Design review of the part built by this model. Coordinates are the model's own, in mm. A direction names the side the tool comes from. Round coordinates to 2 decimals unless told otherwise and drop trailing zeros. Loops run counter-clockwise (first coordinate to the right, second up) from the corner with the lowest first, then second, coordinate; pieces in that order, holes last. Notation, with made-up numbers: (-15.75, -31) -> (-0.75, -31) arc R13 ccw to (-0.75, -16) -> close; hole circle Ø3 at (58, -23.75). An arc over 180 degrees is marked (long way). Use a Markdown table: item, result. Add a question column.
from build123d import *
from build123d.topology import SkipClean

# Parameters (mm, degrees)
SKETCH1_R           = 2.875
SKETCH1_W           = 55.75
SKETCH1_H           = 3.25
BOSS_EXTRUDE1_DEPTH = 3.25
SKETCH1_4_W         = 55.75
SKETCH1_4_H         = 3.25
BOSS_EXTRUDE2_DEPTH = 40
CUT_EXTRUDE2_DEPTH  = 43.25
BOSS_EXTRUDE4_DEPTH = 2
BOSS_EXTRUDE5_DEPTH = 43.25
SKETCH2_R           = 5
SKETCH2_R_2         = 2.875
CUT_EXTRUDE1_DEPTH  = 17.25
FILLET1_R           = 1
SKETCH2_3_R         = 5
SKETCH2_3_R_2       = 2.875
BOSS_EXTRUDE6_DEPTH = 3.25
SKETCH4_R           = 1.5
CUT_EXTRUDE4_DEPTH  = 45.25
FILLET4_R           = 1
FILLET5_R           = 10


# Some blends are built 0.0001 mm under size
with BuildPart() as part:
    # Sketch1 → Boss-Extrude1 (new body)
    # profile 1 of 2: a face of its own
    with BuildSketch(Plane.XY):
        Polygon((-17.875, -10), (37.875, -10), (37.875, -6.375), (37.875, 26.375), (-17.875, 26.375), (-17.875, -6.375), align=None)
        with Locations(Location((20, 20, 0), (0, 0, 180))):
            Circle(SKETCH1_R, mode=Mode.SUBTRACT)
        with Locations(Location((20, 0, 0), (0, 0, 180))):
            Circle(SKETCH1_R, mode=Mode.SUBTRACT)
        with Locations(Location((0, 0, 0), (0, 0, 180))):
            Circle(SKETCH1_R, mode=Mode.SUBTRACT)
        with Locations(Location((0, 20, 0), (0, 0, 180))):
            Circle(SKETCH1_R, mode=Mode.SUBTRACT)
    # profile 2 of 2: a face of its own
    with BuildSketch(Plane.XY):
        with Locations((10, -11.625)):
            Rectangle(SKETCH1_W, SKETCH1_H)
    extrude(amount=BOSS_EXTRUDE1_DEPTH)

    # Sketch1<4> → Boss-Extrude2 (add)
    with BuildSketch(Plane.XY):
        with Locations((10, -11.625)):
            Rectangle(SKETCH1_4_W, SKETCH1_4_H)
    extrude(amount=-BOSS_EXTRUDE2_DEPTH)

    # Sketch3 → Cut-Extrude2 (cut)
    with BuildSketch(Plane.XY.offset(3.25)):
        with BuildLine():
            Line((12.253469547, -13.25), (7.746530453, -13.25))
            ThreePointArc((7.746530453, -13.25), (7.84573728, -20.807857289), (14.375, -17))
            ThreePointArc((14.375, -17), (13.807857289, -14.84573728), (12.253469547, -13.25))
        make_face()
        with BuildLine():
            ThreePointArc((12.253469547, -13.25), (10, -12.625), (7.746530453, -13.25))
            Line((7.746530453, -13.25), (12.253469547, -13.25))
        make_face()
    extrude(amount=-CUT_EXTRUDE2_DEPTH, mode=Mode.SUBTRACT)

    # Sketch3<4> → Boss-Extrude4 (add)
    with BuildSketch(Plane.XY.offset(3.25)):
        Polygon((3.793484606, -13.25), (-17.875, -13.25), (-17.875, -27.25), (37.875, -27.25), (37.875, -13.25), (16.206515394, -13.25), (18.371578903, -17), (14.185789452, -24.25), (5.814210548, -24.25), (1.628421097, -17), align=None)
        Polygon((37.875, -6.75), (-17.875, -6.75), (-17.875, -13.25), (3.793484606, -13.25), (5.814210548, -9.75), (14.185789452, -9.75), (16.206515394, -13.25), (37.875, -13.25), align=None)
    extrude(amount=BOSS_EXTRUDE4_DEPTH)

    # Sketch3<5> → Boss-Extrude5 (add)
    with SkipClean():  # the faces are left unmerged after this step: merging them gives an invalid solid
        with BuildSketch(Plane.XY.offset(3.25)):
            Polygon((3.793484606, -13.25), (-17.875, -13.25), (-17.875, -27.25), (37.875, -27.25), (37.875, -13.25), (16.206515394, -13.25), (18.371578903, -17), (14.185789452, -24.25), (5.814210548, -24.25), (1.628421097, -17), align=None)
            with BuildLine():
                Line((7.746530453, -13.25), (3.793484606, -13.25))
                Line((3.793484606, -13.25), (1.628421097, -17))
                Line((1.628421097, -17), (5.814210548, -24.25))
                Line((5.814210548, -24.25), (14.185789452, -24.25))
                Line((14.185789452, -24.25), (18.371578903, -17))
                Line((18.371578903, -17), (16.206515394, -13.25))
                Line((16.206515394, -13.25), (12.253469547, -13.25))
                ThreePointArc((12.253469547, -13.25), (13.807857289, -14.84573728), (14.375, -17))
                ThreePointArc((14.375, -17), (7.84573728, -20.807857289), (7.746530453, -13.25))
            make_face()
        extrude(amount=-BOSS_EXTRUDE5_DEPTH)

    # Sketch2 → Cut-Extrude1 (cut)
    # profile 1 of 8: a face of its own
    with SkipClean():  # the faces are left unmerged after this step: merging them gives an invalid solid
        with BuildSketch(Plane.XZ.offset(10)):
            with Locations(Location((20, -10, 0), (0, 0, 90))):
                Circle(SKETCH2_R)
            with Locations((20, -10)):
                Circle(SKETCH2_R_2, mode=Mode.SUBTRACT)
        # profile 2 of 8: a face of its own
        with BuildSketch(Plane.XZ.offset(10)):
            with Locations((20, -10)):
                Circle(SKETCH2_R_2)
        # profile 3 of 8: a face of its own
        with BuildSketch(Plane.XZ.offset(10)):
            with Locations(Location((0, -10, 0), (0, 0, 90))):
                Circle(SKETCH2_R)
            with Locations((0, -10)):
                Circle(SKETCH2_R_2, mode=Mode.SUBTRACT)
        # profile 4 of 8: a face of its own
        with BuildSketch(Plane.XZ.offset(10)):
            with Locations((0, -10)):
                Circle(SKETCH2_R_2)
        # profile 5 of 8: a face of its own
        with BuildSketch(Plane.XZ.offset(10)):
            with Locations(Location((0, -30, 0), (0, 0, 90))):
                Circle(SKETCH2_R)
            with Locations((0, -30)):
                Circle(SKETCH2_R_2, mode=Mode.SUBTRACT)
        # profile 6 of 8: a face of its own
        with BuildSketch(Plane.XZ.offset(10)):
            with Locations((0, -30)):
                Circle(SKETCH2_R_2)
        # profile 7 of 8: a face of its own
        with BuildSketch(Plane.XZ.offset(10)):
            with Locations(Location((20, -30, 0), (0, 0, 90))):
                Circle(SKETCH2_R)
            with Locations((20, -30)):
                Circle(SKETCH2_R_2, mode=Mode.SUBTRACT)
        # profile 8 of 8: a face of its own
        with BuildSketch(Plane.XZ.offset(10)):
            with Locations((20, -30)):
                Circle(SKETCH2_R_2)
        extrude(amount=CUT_EXTRUDE1_DEPTH, mode=Mode.SUBTRACT)

    # Fillet1
    fillet1_edges = [part.edges().sort_by_distance(p)[0] for p in [
        (10, -6.75, 3.25),
    ]]
    fillet(fillet1_edges, radius=FILLET1_R)
    fillet1_2_edges = [part.edges().sort_by_distance(p)[0] for p in [
        (10, -6.75, 5.25),
    ]]
    fillet(fillet1_2_edges, radius=FILLET1_R - 0.0001)  # a hair under: the kernel refuses the full size

    # Sketch2<3> → Boss-Extrude6 (add)
    # profile 1 of 4: a face of its own
    with BuildSketch(Plane.XZ.offset(10)):
        with Locations(Location((20, -10, 0), (0, 0, 90))):
            Circle(SKETCH2_3_R)
        with Locations(Location((20, -10, 0), (0, 0, 90))):
            Circle(SKETCH2_3_R_2, mode=Mode.SUBTRACT)
    # profile 2 of 4: a face of its own
    with BuildSketch(Plane.XZ.offset(10)):
        with Locations(Location((0, -10, 0), (0, 0, 90))):
            Circle(SKETCH2_3_R)
        with Locations(Location((0, -10, 0), (0, 0, 90))):
            Circle(SKETCH2_3_R_2, mode=Mode.SUBTRACT)
    # profile 3 of 4: a face of its own
    with BuildSketch(Plane.XZ.offset(10)):
        with Locations(Location((0, -30, 0), (0, 0, 90))):
            Circle(SKETCH2_3_R)
        with Locations(Location((0, -30, 0), (0, 0, 90))):
            Circle(SKETCH2_3_R_2, mode=Mode.SUBTRACT)
    # profile 4 of 4: a face of its own
    with BuildSketch(Plane.XZ.offset(10)):
        with Locations(Location((20, -30, 0), (0, 0, 90))):
            Circle(SKETCH2_3_R)
        with Locations(Location((20, -30, 0), (0, 0, 90))):
            Circle(SKETCH2_3_R_2, mode=Mode.SUBTRACT)
    extrude(amount=BOSS_EXTRUDE6_DEPTH)

    # Sketch4 → Cut-Extrude4 (cut)
    with BuildSketch(Plane.XY.offset(5.25)):
        with Locations((33.125, -22.5)):
            Circle(SKETCH4_R)
        with Locations((-13.125, -22.5)):
            Circle(SKETCH4_R)
        with Locations((-13.125, -14.5)):
            Circle(SKETCH4_R)
        with Locations((33.125, -14.5)):
            Circle(SKETCH4_R)
    extrude(amount=-CUT_EXTRUDE4_DEPTH, mode=Mode.SUBTRACT)

    # Fillet4
    fillet4_edges = [part.edges().sort_by_distance(p)[0] for p in [
        (3.721315823, -13.375, 5.25),
        (10, -9.75, 5.25),
        (16.278684177, -13.375, 5.25),
        (16.278684177, -20.625, 5.25),
        (10, -24.25, 5.25),
        (3.721315823, -20.625, 5.25),
    ]]
    fillet(fillet4_edges, radius=FILLET4_R)

    # Fillet5
    # the kernel refuses this fillet: 10 mm, written as the material it takes off along each edge
    with BuildSketch(Plane(origin=(62.875, -10, -40), x_dir=(0, -1, 0), z_dir=(-1, 0, 0))) as fillet5_piece_1:
        with BuildLine():
            CenterArc((FILLET5_R, FILLET5_R), FILLET5_R, 180, 90)
            Line((0, FILLET5_R), (0, 0))
            Line((0, 0), (FILLET5_R, 0))
        make_face()
    extrude(amount=105.75, mode=Mode.SUBTRACT)


solid = part.part
1. Consider section C-C on y = -1.5. State the section outline as (x, z) points (3 decimals), plus the area to 3 significant figures.
2. Insertion check: P1, Ø7.5, axis at x = 0, z = -10, coming from the +Y side; P2, Ø6, axis at x = 18.5, y = 11.5, coming from the -Z side; P3, Ø8, axis at x = 8, y = -8.5, coming from the -Z side. Each pin has a flat end and moves straight along its axis. Give the tip position at first contact, or say it passes through.
3. Mouldability with a two-part tool opening along Z and no side actions: class faces 1 (the face through (10, -24, -40)), 2 (the face through (3.428, -20.718, 4.965)), 3 (the face through (0.623, 22.807, 1.602)), 4 (the face through (-1.5, -20.15, -5.23)) as +Z half, -Z half, draft (parallel to the pull), parting line (faces both ways), or undercut.
4. Consider section A-A on z = -24. State the section outline as (x, y) points (3 decimals), plus the area to 3 significant figures.
5. For faces 5 (the face through (-14.624, -14.434, -16.647)), 6 (the face through (21.101, -11.602, -27.344)), 7 (the face through (16.506, -20.833, 4.965)), 8 (the face through (24.436, -20.152, -7.693)), 9 (the face through (10, 8, 0)), list the 3-axis set-ups (+Z, -Z, +X, -X, +Y, -Y) from which the entire face can be reached by the end or side of a thin tool; tool diameter is ignored.
6. To check wall thickness, follow probe 1 along Y at (x, z) = (20, 2.55) (3 decimals); probe 2 along Z at (x, y) = (20, -21); probe 3 along X at (y, z) = (20, 1) (3 decimals). State the ranges of each line that lie inside material, in increasing order. Write a range as from..to.
7. Consider section D-D on y = -22.5. Give the number of separate pieces and of enclosed holes in the cut face, plus the area to 3 significant figures.
Verdict:
| question | item | result |
|---|---|---|
| 1 | outline | (-17.875, 0) -> (-2.453, 0) -> (-2.453, 3.25) -> (-17.875, 3.25) -> close; (2.453, 0) -> (17.547, 0) -> (17.547, 3.25) -> (2.453, 3.25) -> close; (22.453, 0) -> (37.875, 0) -> (37.875, 3.25) -> (22.453, 3.25) -> close |
| 1 | area | 149 mm² |
| 2 | P1 | stops at y = -10 |
| 2 | P2 | stops at z = 0 |
| 2 | P3 | stops at z = -36.61 |
| 3 | face 1 | -Z half |
| 3 | face 2 | +Z half |
| 3 | face 3 | draft |
| 3 | face 4 | undercut |
| 4 | outline | (-17.875, -27.25) -> (37.875, -27.25) -> (37.875, -10) -> (-17.875, -10) -> close; hole circle Ø3 at (-13.125, -22.5); hole circle Ø3 at (-13.125, -14.5); hole circle Ø8.75 at (10, -17); hole circle Ø3 at (33.125, -22.5); hole circle Ø3 at (33.125, -14.5) |
| 4 | area | 873 mm² |
| 5 | face 5 | +Z, -Z |
| 5 | face 6 | +Y, -Y |
| 5 | face 7 | +Z |
| 5 | face 8 | -Y |
| 5 | face 9 | -Z, +X, -X, +Y |
| 6 | probe 1 | y = -27.25..-2.875, 2.875..17.125, 22.875..26.375 |
| 6 | probe 2 | z = -40..-35, -25..-15, -5..5.25 |
| 6 | probe 3 | x = -17.875..-2.875, 2.875..17.125, 22.875..37.875 |
| 7 | separate pieces | 3 |
| 7 | enclosed holes | 4 |
| 7 | area | 1,920 mm² |
